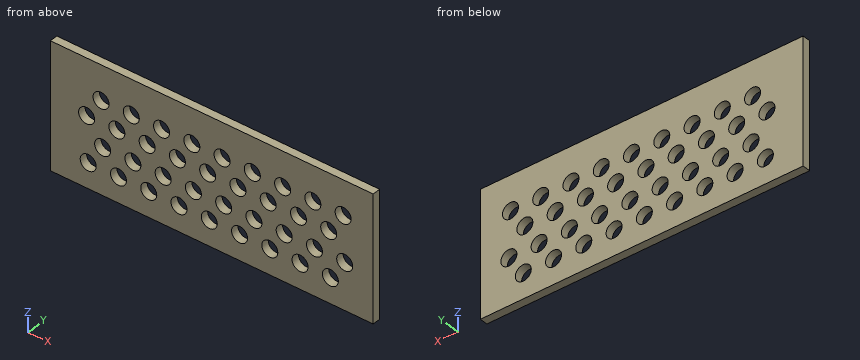
```python
from build123d import *

# Parameters (mm, degrees)
SKETCH1_W           = 128
SKETCH1_H           = 50
BOSS_EXTRUDE1_DEPTH = 3.175
SKETCH2_R           = 3.175
CUT_EXTRUDE1_DEPTH  = 3.175


with BuildPart() as part:
    # Sketch1 → Boss-Extrude1 (new body)
    with BuildSketch(Plane(origin=(0, 0, 0), x_dir=(1, 0, 0), z_dir=(0, 1, 0))):
        with Locations((7.729468599, 5.299516908)):
            Rectangle(SKETCH1_W, SKETCH1_H)
    extrude(amount=BOSS_EXTRUDE1_DEPTH)

    # Sketch2 → Cut-Extrude1 (cut)
    with BuildSketch(Plane(origin=(0, 3.175, 0), x_dir=(1, 0, 0), z_dir=(0, 1, 0))):
        with Locations((-41.270531401, 20.299516908)):
            Circle(SKETCH2_R)
        with Locations((-29.270531401, 20.299516908)):
            Circle(SKETCH2_R)
        with Locations((-17.270531401, 20.299516908)):
            Circle(SKETCH2_R)
        with Locations((-5.270531401, 20.299516908)):
            Circle(SKETCH2_R)
        with Locations((6.729468599, 20.299516908)):
            Circle(SKETCH2_R)
        with Locations((18.729468599, 20.299516908)):
            Circle(SKETCH2_R)
        with Locations((30.729468599, 20.299516908)):
            Circle(SKETCH2_R)
        with Locations((42.729468599, 20.299516908)):
            Circle(SKETCH2_R)
        with Locations((54.729468599, 20.299516908)):
            Circle(SKETCH2_R)
        with Locations((-35.558058134, 11.846734249)):
            Circle(SKETCH2_R)
        with Locations((-23.558058134, 11.846734249)):
            Circle(SKETCH2_R)
        with Locations((-11.558058134, 11.846734249)):
            Circle(SKETCH2_R)
        with Locations((0.441941866, 11.846734249)):
            Circle(SKETCH2_R)
        with Locations((12.441941866, 11.846734249)):
            Circle(SKETCH2_R)
        with Locations((24.441941866, 11.846734249)):
            Circle(SKETCH2_R)
        with Locations((36.441941866, 11.846734249)):
            Circle(SKETCH2_R)
        with Locations((48.441941866, 11.846734249)):
            Circle(SKETCH2_R)
        with Locations((60.441941866, 11.846734249)):
            Circle(SKETCH2_R)
        with Locations((-41.90349241, 2.495409821)):
            Circle(SKETCH2_R)
        with Locations((-29.90349241, 2.495409821)):
            Circle(SKETCH2_R)
        with Locations((-17.90349241, 2.495409821)):
            Circle(SKETCH2_R)
        with Locations((-5.90349241, 2.495409821)):
            Circle(SKETCH2_R)
        with Locations((6.09650759, 2.495409821)):
            Circle(SKETCH2_R)
        with Locations((18.09650759, 2.495409821)):
            Circle(SKETCH2_R)
        with Locations((30.09650759, 2.495409821)):
            Circle(SKETCH2_R)
        with Locations((42.09650759, 2.495409821)):
            Circle(SKETCH2_R)
        with Locations((54.09650759, 2.495409821)):
            Circle(SKETCH2_R)
        with Locations((-36.191019143, -5.957372838)):
            Circle(SKETCH2_R)
        with Locations((-24.191019143, -5.957372838)):
            Circle(SKETCH2_R)
        with Locations((-12.191019143, -5.957372838)):
            Circle(SKETCH2_R)
        with Locations((-0.191019143, -5.957372838)):
            Circle(SKETCH2_R)
        with Locations((11.808980857, -5.957372838)):
            Circle(SKETCH2_R)
        with Locations((23.808980857, -5.957372838)):
            Circle(SKETCH2_R)
        with Locations((35.808980857, -5.957372838)):
            Circle(SKETCH2_R)
        with Locations((47.808980857, -5.957372838)):
            Circle(SKETCH2_R)
        with Locations((59.808980857, -5.957372838)):
            Circle(SKETCH2_R)
    extrude(amount=-CUT_EXTRUDE1_DEPTH, mode=Mode.SUBTRACT)


solid = part.part
```
For this review, take the finished solid that the model builds, in its own axes (mm). Coordinates: 2 decimals unless noted, no trailing zeros. Answer in a Markdown table with one row per item. Add a question column.
Q1. For probe 1 along Z at (x, y) = (30.5, 1.1); probe 2 along Z at (x, y) = (21, 0.65); probe 3 along Z at (x, y) = (-35, 1.65), list the stretches that pass through material, from the lowest coordinate up.
Q2. We need section A-A, the plane y = 1.75. Count the separate pieces of the cut face and the enclosed holes in it, and give its area (3 significant figures).
Q3. For P1, Ø8.5, axis at x = -5.27, z = -20.3, coming from the -Y side; P2, Ø4, axis at x = -23.56, z = -11.85, coming from the -Y side (3 decimals), all flat-tipped, find the tip position at first contact; note any pin that passes through.
Answer list:
| question | item | result |
|---|---|---|
| 1 | probe 1 | z = -30.3 to -23.47, -17.13 to -5.64, 0.65 to 19.7 |
| 1 | probe 2 | z = -30.3 to -22.52, -18.08 to -3.78, -1.21 to 4.48, 7.44 to 19.7 |
| 1 | probe 3 | z = -30.3 to -14.97, -8.72 to 3.01, 8.9 to 19.7 |
| 2 | separate pieces | 1 |
| 2 | enclosed holes | 36 |
| 2 | area | 5,260 mm2 |
| 3 | P1 | stops at y = 0 |
| 3 | P2 | passes through |
